from build123d import *

# Parameters (mm, degrees)
SKETCH_W            = 1200
SKETCH_H            = 500
PAD_DEPTH           = 18
SKETCH006_W         = 200
SKETCH006_H         = 200
POCKET_DEPTH        = 18
LINEARPATTERN_COUNT = 4
LINEARPATTERN_PITCH = 280


with BuildPart() as part:
    # Sketch → Pad (new body)
    with BuildSketch(Plane.XY):
        Rectangle(SKETCH_W, SKETCH_H)
    extrude(amount=PAD_DEPTH)

    # Sketch006 (on Face6 of Pad) → Pocket (cut)
    with BuildSketch(Plane.XY.offset(18)):
        with Locations((-420, 0)):
            Rectangle(SKETCH006_W, SKETCH006_H)
    pocket = extrude(amount=-POCKET_DEPTH, mode=Mode.SUBTRACT)

    # LinearPattern: Pocket ×4
    with Locations(*[(i * LINEARPATTERN_PITCH, 0, 0) for i in range(1, LINEARPATTERN_COUNT)]):
        add(pocket, mode=Mode.SUBTRACT)


solid = part.part
The listing builds one solid part. Answer for the finished solid, in the listing's coordinates (mm). Give positions to 0.01 mm unless a question says otherwise; leave off trailing zeros. Loops run counter-clockwise (first coordinate to the right, second up) from the corner with the lowest first, then second, coordinate; pieces in that order, holes last. Notation, with made-up numbers: (87, 11.25) - (101, 11.25) arc R16 ccw to (101, 19.25) - close; hole circle Ø3 at (49.5, 7.25). An arc over 180 degrees is marked (long way). Use one line per item in the form item = value.
1. Section A-A on x = -190.5 is taken. Give the vertices of the cut face in (y, z).
Calculated:
outline = (-250, 0) - (-100, 0) - (-100, 18) - (-250, 18) - close; (100, 0) - (250, 0) - (250, 18) - (100, 18) - close
2. Find the intervals of material crossed by line 1 along X through (y, z) = (-71.5, 3.25); line 2 along Y through (x, z) = (172.5, 1), in increasing order. Write a range as [from, to].
Calculated:
line_1 = [-600, -520], [-320, -240], [-40, 40], [240, 320], [520, 600]
line_2 = [-250, -100], [100, 250]
3. Section B-B on y = -76 is taken. Give the vertices of the cut face in (x, z).
Calculated:
outline = (-600, 0) - (-520, 0) - (-520, 18) - (-600, 18) - close; (-320, 0) - (-240, 0) - (-240, 18) - (-320, 18) - close; (-40, 0) - (40, 0) - (40, 18) - (-40, 18) - close; (240, 0) - (320, 0) - (320, 18) - (240, 18) - close; (520, 0) - (600, 0) - (600, 18) - (520, 18) - close
4. Section C-C on z = 8 is taken. Give the vertices of the cut face in (x, y).
Calculated:
outline = (-600, -250) - (600, -250) - (600, 250) - (-600, 250) - close; hole (-520, -100) - (-320, -100) - (-320, 100) - (-520, 100) - close; hole (-240, -100) - (-40, -100) - (-40, 100) - (-240, 100) - close; hole (40, -100) - (240, -100) - (240, 100) - (40, 100) - close; hole (320, -100) - (520, -100) - (520, 100) - (320, 100) - close
